The model under review builds one solid part; all positions refer to its coordinate system, in mm. A direction names the side the tool comes from. Round coordinates to 2 decimals unless told otherwise and drop trailing zeros. Order: outer loops, then holes, each group sorted by start corner. A loop starts at its lowest first (then second) coordinate and runs counter-clockwise, first axis right, second up. Notation, with made-up numbers: M -1.75,-34.5 L 45.25,-34.5 A28 ccw 45.25,3.5 Z; hole C 84,-15.75 d1. An arc over 180 degrees is marked long. Answer as a JSON object with one key per item and string values. Group by question number.
1) To check wall thickness, follow line 1 (Z direction, x = 0.75, y = 55.25); line 2 (X direction, y = 52.5, z = -7); line 3 (Y direction, x = 0.25, z = -4). State the ranges of each line that lie inside material, in increasing order.
2) Consider section A-A, the plane z = -6.75. Write out the cut boundary in (x, y) (3 decimals).
3) Insertion check: pin 1 Ø1.5 at (y, z) = (50.5, -1.5) entering from -X; pin 2 Ø4 at (x, y) = (0, 49.5) entering from -Z (3 decimals); pin 3 Ø5 at (y, z) = (49.5, -1.5) entering from -X. Each pin has a flat end and moves straight along its axis. Give the tip position at first contact, or say it passes through.
4) For faces 4 (the cylindrical face through (-0.638, 57.783, 1.486)), 5 (the flat face through (2, 51, 0)), list the 3-axis set-ups (+Z, -Z, +X, -X, +Y, -Y) from which the entire face can be reached by the end or side of a thin tool; tool diameter is ignored.
5) The part is to be moulded in two halves that separate along X. For faces 1 (the cylindrical face through (-0.07, 53.42, -2.93)), 2 (the cylindrical face through (-0.25, 54.81, -4.46)), 3 (the flat face through (0, 52, 3)), say which applies: +X half, -X half, draft (parallel to the pull), parting line (faces both ways), or undercut.
```python
from build123d import *

# Parameters (mm, degrees)
SKETCH1_R           = 4.9
SKETCH1_R_2         = 1.9
BOSS_EXTRUDE1_DEPTH = 3
SKETCH1_4_R         = 1.9
BOSS_EXTRUDE2_DEPTH = 9.03
FILLET1_R           = 0.5
CHAMFER1_SIZE       = 0.5
CUT_EXTRUDE1_REACH  = 14.03
SKETCH2_R           = 0.5


with BuildPart() as part:
    # Sketch1 → Boss-Extrude1 (new body)
    with BuildSketch(Plane.XY):
        with Locations((-1.7071e-05, 52.925001209)):
            Circle(SKETCH1_R)
        with Locations((-1.7071e-05, 52.925001209)):
            Circle(SKETCH1_R_2, mode=Mode.SUBTRACT)
        with Locations((-1.7071e-05, 52.925001209)):
            Circle(SKETCH1_R_2)
    extrude(amount=BOSS_EXTRUDE1_DEPTH)

    # Sketch1<4> → Boss-Extrude2 (add)
    with BuildSketch(Plane.XY):
        with Locations((-1.7071e-05, 52.925001209)):
            Circle(SKETCH1_4_R)
    extrude(amount=-BOSS_EXTRUDE2_DEPTH)

    # Fillet1
    fillet1_edges = [part.edges().sort_by_distance(p)[0] for p in [
        (-1.900017071, 52.925001209, 0),
    ]]
    fillet(fillet1_edges, radius=FILLET1_R)

    # Chamfer1
    chamfer1_edges = [part.edges().sort_by_distance(p)[0] for p in [
        (-4.900017071, 52.925001209, 3),
        (-1.900017071, 52.925001209, -9.03),
        (-4.900017071, 52.925001209, 0),
    ]]
    chamfer(chamfer1_edges, length=CHAMFER1_SIZE)

    # Sketch2 → Cut-Extrude1 (cut, up to next)
    with BuildSketch(Plane.XY.offset(3), mode=Mode.PRIVATE) as cut_extrude1_sk1:
        with Locations((-1.7071e-05, 52.925001209)):
            Circle(SKETCH2_R)
    cut_extrude1_tool1 = extrude(cut_extrude1_sk1.sketch, amount=-CUT_EXTRUDE1_REACH, mode=Mode.PRIVATE) & part.part
    add(cut_extrude1_tool1.solids().sort_by_distance((-1.7e-05, 52.925001, 3))[0], mode=Mode.SUBTRACT)


solid = part.part
```
Results list:
{
 "1": {"line 1": "0 to 3", "line 2": "-1.85 to -0.26, 0.26 to 1.85", "line 3": "51.04 to 52.49, 53.36 to 54.81"},
 "2": {"outline": "C 0,52.925 d3.8; hole C 0,52.925 d1"},
 "3": {"pin 1": "x = -0.9", "pin 2": "z = -9.005", "pin 3": "x = -4.51"},
 "4": {"face 4": "+Z, -Z", "face 5": "-Z"},
 "5": {"face 1": "undercut", "face 2": "parting line", "face 3": "draft"}
}
